Design review of the part built by this model. Coordinates are the model's own, in mm. A direction names the side the tool comes from. Round coordinates to 2 decimals unless told otherwise and drop trailing zeros. Order: outer loops, then holes, each group sorted by start corner. A loop starts at its lowest first (then second) coordinate and runs counter-clockwise, first axis right, second up.
from build123d import *

# Parameters (mm, degrees)
EXTRUDE_1_DEPTH     = 18
SKETCH_2_W          = 14
SKETCH_2_H          = 26
CUT_EXTRUDE_1_DEPTH = 18
CUT_EXTRUDE_2_DEPTH = 18
SKETCH_4_R          = 3
CUT_EXTRUDE_3_DEPTH = 18


with BuildPart() as part:
    # 스케치1 → 보스-돌출1 (new body)
    with BuildSketch(Plane(origin=(0, 0, 0), x_dir=(0, 0, -1), z_dir=(1, 0, 0))):
        Polygon((0, 0), (20, 0), (20, 2), (2, 28), (0, 28), align=None)
    extrude(amount=EXTRUDE_1_DEPTH)

    # 스케치2 → 컷-돌출1 (cut)
    with BuildSketch(Plane(origin=(0, 0, -20), x_dir=(-1, 0, 0), z_dir=(0, 0, -1))):
        with Locations((-9, 15)):
            Rectangle(SKETCH_2_W, SKETCH_2_H)
    extrude(amount=-CUT_EXTRUDE_1_DEPTH, mode=Mode.SUBTRACT)

    # 스케치3 → 컷-돌출2 (cut)
    with BuildSketch(Plane(origin=(0, 0, -2), x_dir=(-1, 0, 0), z_dir=(0, 0, -1))):
        with BuildLine():
            Line((-6, 23), (-6, 7))
            ThreePointArc((-6, 7), (-9, 4), (-12, 7))
            Line((-12, 7), (-12, 23))
            ThreePointArc((-12, 23), (-9, 26), (-6, 23))
        make_face()
    extrude(amount=-CUT_EXTRUDE_2_DEPTH, mode=Mode.SUBTRACT)

    # 스케치4 → 컷-돌출3 (cut)
    with BuildSketch(Plane(origin=(0, 2, 0), x_dir=(1, 0, 0), z_dir=(0, 1, 0))):
        with Locations(Location((9, 11, 0), (0, 0, 270))):
            Circle(SKETCH_4_R)
    extrude(amount=-CUT_EXTRUDE_3_DEPTH, mode=Mode.SUBTRACT)


solid = part.part
1) The part is to be moulded in two halves that separate along X. For faces 4 (the face through (18, 11, -8)), 5 (the face through (17, 15, -11)), 6 (the face through (16, 9, -7)), say which applies: released by +X, released by -X, zero draft, split by the parting line, or undercut.
Results:
face 4: released by +X
face 5: zero draft
face 6: undercut
2) For faces 1 (the face through (2, 9, -7)), 2 (the face through (0, 11, -8)), 3 (the face through (12, 15, -1)), list the 3-axis set-ups (+Z, -Z, +X, -X, +Y, -Y) from which the entire face can be reached by the end or side of a thin tool; tool diameter is ignored.
Results:
face 1: -Z, +Y
face 2: +Z, -Z, -X, +Y, -Y
face 3: +Z, -Z
3) Take a section at B-B on z = -11. Give the boundary of the cut face in (x, y).
Results:
outline: (0, 0) - (6, 0) - (6, 2) - (2, 2) - (2, 15) - (0, 15) - close; (12, 0) - (18, 0) - (18, 15) - (16, 15) - (16, 2) - (12, 2) - close
4) Take a section at C-C on y = 21.5. Give the boundary of the cut face in (x, z), plus the area to 3 significant figures.
Results:
outline: (0, -6.5) - (2, -6.5) - (2, -2) - (6, -2) - (6, 0) - (0, 0) - close; (12, -2) - (16, -2) - (16, -6.5) - (18, -6.5) - (18, 0) - (12, 0) - close
area: 42.0 mm2
5) Take a section at D-D on z = -4.25. Give the boundary of the cut face in (x, y), plus the area to 3 significant figures.
Results:
outline: (0, 0) - (18, 0) - (18, 24.75) - (16, 24.75) - (16, 2) - (2, 2) - (2, 24.75) - (0, 24.75) - close
area: 127 mm2
6) To check wall thickness, follow line 1 along X through (y, z) = (1, -11); line 2 along X through (y, z) = (24.5, -2.25); line 3 along Z through (x, y) = (12.75, 26.75). State the ranges of each line that lie inside material, in increasing order.
Results:
line 1: x = 0 to 6, 12 to 18
line 2: x = 0 to 2, 16 to 18
line 3: z = -2 to 0
7) Take a section at A-A on x = 9. Give the boundary of the cut face in (y, z), plus the area to 3 significant figures.
Results:
outline: (0, -20) - (2, -20) - (2, -14) - (0, -14) - close; (0, -8) - (2, -8) - (2, -2) - (4, -2) - (4, 0) - (0, 0) - close; (26, -2) - (28, -2) - (28, 0) - (26, 0) - close
area: 36.0 mm2
8) Clearance check with a flat-ended pin moving along its axis: P1, Ø7, axis at x = 7.5, y = 9, coming from the -Z side. State where the tip first meets the part, or that it passes through.
Results:
P1: stops at z = -2
